CAD build for the part. Positions are in the model's coordinates, mm. Give positions to 0.01 mm unless a question says otherwise; leave off trailing zeros. Loops run counter-clockwise (first coordinate to the right, second up) from the corner with the lowest first, then second, coordinate; pieces in that order, holes last. Notation, with made-up numbers: (-39.5, -14.75) - (-29.5, -14.75) arc R31 cw to (-29.5, 23.25) - close; hole circle Ø11 at (69, 58). An arc over 180 degrees is marked (long way). Return JSON: item names as keys, results as strings.
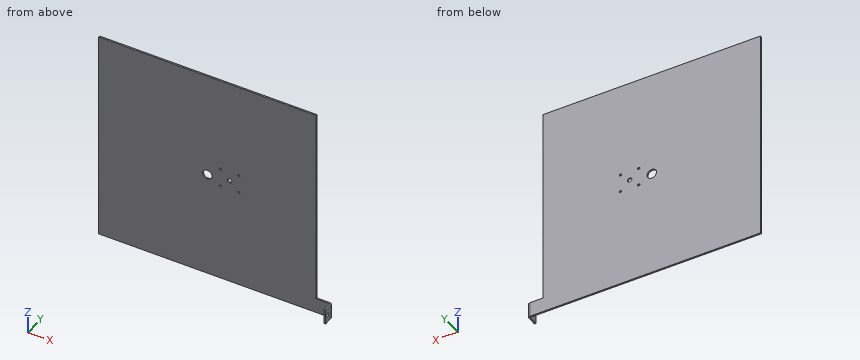
from build123d import *

# Parameters (mm, degrees)
BASE_FLANGE1_DEPTH           = 2.54
SKETCH6_R                    = 3.81
SKETCH6_R_2                  = 1.905
CUT_EXTRUDE1_DEPTH           = 2.54
SKETCH7_R                    = 8
CUT_EXTRUDE2_DEPTH           = 2.54
EDGE_FLANGE1_STRIP_W         = 11.6332
EDGE_FLANGE1_STRIP_H         = 2.54
EDGE_FLANGE1_STRIP_CUT_DEPTH = 25.4
EDGE_FLANGE1_DEPTH           = 25.4
SKETCH12_R                   = 3.302
CUT_EXTRUDE3_DEPTH           = 2.54


# Sheet-metal steps are written as plain solids
with BuildPart() as part:
    # Sketch1 → Base-Flange1 (new body)
    with BuildSketch(Plane(origin=(0, 0, 0), x_dir=(1, 0, 0), z_dir=(0, 1, 0))):
        Polygon((0, 0), (368.3, 0), (368.3, 342.9), (394.208, 342.9), (394.208, 368.3), (368.3, 368.3), (0, 368.3), align=None)
    extrude(amount=-BASE_FLANGE1_DEPTH)

    # Sketch6 → Cut-Extrude1 (cut)
    with BuildSketch(Plane(origin=(0, 0, 0), x_dir=(1, 0, 0), z_dir=(0, 1, 0))):
        with Locations(Location((221.844041513, 180.737580342, 0), (0, 0, 270))):
            Circle(SKETCH6_R)
        with Locations(Location((237.338041513, 165.243580342, 0), (0, 0, 270))):
            Circle(SKETCH6_R_2)
        with Locations(Location((237.338041513, 196.231580342, 0), (0, 0, 270))):
            Circle(SKETCH6_R_2)
        with Locations(Location((206.350041513, 196.231580342, 0), (0, 0, 270))):
            Circle(SKETCH6_R_2)
        with Locations(Location((206.350041513, 165.243580342, 0), (0, 0, 270))):
            Circle(SKETCH6_R_2)
    extrude(amount=-CUT_EXTRUDE1_DEPTH, mode=Mode.SUBTRACT)

    # Sketch7 → Cut-Extrude2 (cut)
    with BuildSketch(Plane(origin=(0, -2.54, 0), x_dir=(-1, 0, 0), z_dir=(0, -1, 0))):
        with Locations(Location((-184.15, 184.15, 0), (0, 0, 90))):
            Circle(SKETCH7_R)
    extrude(amount=-CUT_EXTRUDE2_DEPTH, mode=Mode.SUBTRACT)

    # Edge-Flange1 strip (across the edge) → Edge-Flange1 strip cut (cut)
    with BuildSketch(Plane(origin=(394.208, -2.54, -368.3), x_dir=(-1, 0, 0), z_dir=(0, 0, 1))):
        with Locations((-2.54, -1.27)):
            Rectangle(EDGE_FLANGE1_STRIP_W, EDGE_FLANGE1_STRIP_H)
    extrude(amount=EDGE_FLANGE1_STRIP_CUT_DEPTH, mode=Mode.SUBTRACT)

    # Edge-Flange1 section (across the edge) → Edge-Flange1 (add)
    with BuildSketch(Plane(origin=(394.208, -2.54, -368.3), x_dir=(-1, 0, 0), z_dir=(0, 0, 1))):
        with BuildLine():
            Line((0, 0.7366), (0, 16.51))
            Line((0, 16.51), (2.54, 16.51))
            Line((2.54, 16.51), (2.54, 0.7366))
            ThreePointArc((2.54, 0.7366), (2.755745145, 0.215745145), (3.2766, 0))
            Line((3.2766, 0), (3.2766, -2.54))
            ThreePointArc((3.2766, -2.54), (0.959693921, -1.580306079), (0, 0.7366))
        make_face()
    extrude(amount=EDGE_FLANGE1_DEPTH)

    # Sketch12 → Cut-Extrude3 (cut)
    with BuildSketch(Plane(origin=(394.208, 0, 0), x_dir=(0, 0, -1), z_dir=(1, 0, 0))):
        with Locations(Location((355.6, -12.7, 0), (0, 0, 90))):
            Circle(SKETCH12_R)
    extrude(amount=-CUT_EXTRUDE3_DEPTH, mode=Mode.SUBTRACT)


solid = part.part
1. Cut at B-B, the plane x = 184.15. Write the cut outline in (y, z), plus the area to 3 significant figures.
Values follow:
{"outline": "(-2.54, -368.3) - (0, -368.3) - (0, -192.15) - (-2.54, -192.15) - close; (-2.54, -176.15) - (0, -176.15) - (0, 0) - (-2.54, 0) - close", "area": "895 mm²"}
2. Drop flat-ended pins along their axis: P1, Ø6, axis at x = 237.34, z = -196.23, coming from the -Y side; P2, Ø7.5, axis at y = -12.7, z = -355.6, coming from the +X side; P3, Ø8, axis at y = -9, z = -350.5, coming from the -X side; P4, Ø3, axis at y = -1, z = -174.5, coming from the +X side. Give the stop position or say it passes through.
Values follow:
{"P1": "stops at y = -2.54", "P2": "stops at x = 394.21", "P3": "stops at x = 391.67", "P4": "stops at x = 368.3"}
3. Cut at D-D, the plane z = -325. Write the cut outline in (x, y), plus the area to 3 significant figures.
Values follow:
{"outline": "(0, -2.54) - (368.3, -2.54) - (368.3, 0) - (0, 0) - close", "area": "935 mm²"}
4. Cut at A-A, the plane y = -12.7. Write the cut outline in (x, z), plus the area to 3 significant figures.
Values follow:
{"outline": "(391.67, -368.3) - (394.21, -368.3) - (394.21, -358.9) - (391.67, -358.9) - close; (391.67, -352.3) - (394.21, -352.3) - (394.21, -342.9) - (391.67, -342.9) - close", "area": "47.7 mm²"}
5. Cut at C-C, the plane x = 59. Write the cut outline in (y, z), plus the area to 3 significant figures.
Values follow:
{"outline": "(-2.54, -368.3) - (0, -368.3) - (0, 0) - (-2.54, 0) - close", "area": "935 mm²"}
6. Drill centre lines: probe 1 along Z at (x, y) = (392.9, -12.7); probe 2 along Y at (x, z) = (319, -45); probe 3 along X at (y, z) = (-2.25, -315.5). Where is each one in solid material? Low to high.
Values follow:
{"probe 1": "z = -368.3 to -358.9, -352.3 to -342.9", "probe 2": "y = -2.54 to 0", "probe 3": "x = 0 to 368.3"}
